Solid Edge part; units mm, degrees
sketch "Sketch1" plane through (0, 0, 0) normal (0, -1, 0) x (1, 0, 0)
  line L0 (-70, 127) -> (-70, 68.5)
  line L1 (-70, 68.5) -> (-65, 68.5)
  line L2 (-65, 68.5) -> (-65, 63.5)
  line L3 (-65, 63.5) -> (-55, 63.5)
  line L4 (-55, 63.5) -> (-55, 68.5)
  line L5 (-55, 68.5) -> (-60, 68.5)
  line L6 (-60, 68.5) -> (-60, 73.5)
  line L7 (-60, 73.5) -> (-65, 73.5)
  line L8 (-65, 73.5) -> (-65, 122)
  line L9 (-65, 122) -> (65, 122)
  line L10 (65, 122) -> (65, 73.5)
  line L11 (65, 73.5) -> (60, 73.5)
  line L12 (60, 73.5) -> (60, 68.5)
  line L13 (60, 68.5) -> (55, 68.5)
  line L14 (55, 68.5) -> (55, 63.5)
  line L15 (55, 63.5) -> (65, 63.5)
  line L16 (65, 63.5) -> (65, 68.5)
  line L17 (65, 68.5) -> (70, 68.5)
  line L18 (70, 68.5) -> (70, 127)
  line L19 (70, 127) -> (-70, 127)
  dimension "D1" = 65
  dimension "D2" = 55
  dimension "D3" = 60
  dimension "D4" = 55
  dimension "D5" = 55
  dimension "D6" = 60
  dimension "D7" = 65
  dimension "D8" = 60
  dimension "D9" = 65
revolve "RevolvedProtrusion1" add sketch "Sketch1" angle 360 about axis through (-79.3986, 0, 0) along (1, 0, 0)
fillet "Round1" radius 5 4 edges at (-65, 0, -122) (-70, 0, -127) (65, 0, -122) (70, 0, -127)
properties material "Phenolic"
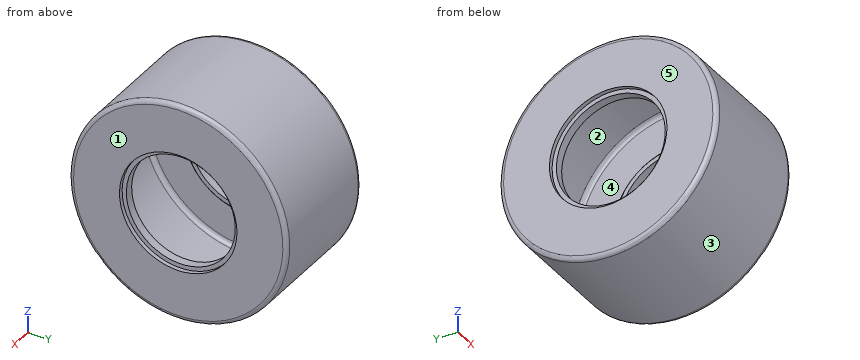
The listing builds one solid part. Answer for the finished solid, in the listing's coordinates (mm). Face numbers are marked on the shaded views. A direction names the side the tool comes from. Coordinates: 2 decimals unless noted, no trailing zeros. Write each loop counter-clockwise with the first axis right and the second up, starting at its lowest first coordinate (ties: lowest second). Pieces come first, ordered by that corner, then holes. Notation, with made-up numbers: M -4,56.5 L 8,56.5 A22 ccw 8,76.5 Z; hole C 3.25,0.5 d6. An arc over 180 degrees is marked long. Write each question's results on one line, items separated by ' | '.
Item 1: Which of the six approach directions +Z, -Z, +X, -X, +Y, -Y give full straight-line access (tool end or side, diameter ignored) to the marked faces 1 and 2?
Answer below:
face 1: +Z, -Z, +X, +Y, -Y | face 2: none
Item 2: Consider probe 1 along Y at (x, z) = (-57.75, 0); probe 2 along X at (y, z) = (10, 78); probe 3 along Z at (x, y) = (32.5, 0). Determine where each line is inside the solid, lowest interval first. Write a range as [from, to].
Answer below:
probe 1: [-127, -122], [-68.5, -63.5], [63.5, 68.5], [122, 127] | probe 2: [-70, -65], [65, 70] | probe 3: [-127, -122], [122, 127]
Item 3: The part is cut by section A-A on x = -51. Determine the outline of the cut face in (y, z).
Answer below:
outline: C 0,0 d254; hole C 0,0 d244
Item 4: For a pull along Y with two mould halves and no side action, classify the marked faces 3, 4 and 5 as released by +Y, released by -Y, zero draft, split by the parting line, or undercut.
Answer below:
face 3: split by the parting line | face 4: undercut | face 5: zero draft
Item 5: Given P1, Ø8, axis at y = -23, z = -57, coming from the -X side; P2, Ø5, axis at x = 8, y = -33.5, coming from the -Z side; P3, Ø4, axis at x = 49.5, y = -45, coming from the +Z side, each flat-ended and moving along its own axis, determine where each tip first touches the part or whether it passes through.
Answer below:
P1: x = -65 | P2: z = -123.16 | P3: z = 119.5
